Could you check a few things on this model? Use its own coordinates, in mm. Face numbers are marked on the shaded views. Give positions to 0.01 mm unless a question says otherwise; leave off trailing zeros. Order: outer loops, then holes, each group sorted by start corner. A loop starts at its lowest first (then second) coordinate and runs counter-clockwise, first axis right, second up.
(1) If I drill on probe 1 along Y at (x, z) = (121, 39); probe 2 along Z at (x, y) = (59.5, 113.5); probe 3 along X at (y, z) = (58.5, 81), over which ranges is the centre line in solid material (lowest first)?
(2) Imagine slicing it at B-B, the plane x = 42. Write out the boundary of the cut face in (y, z), then the cut area to 3 significant figures.
(3) Will these pins go through, and if not, where does the flat tip stop? pin 1 (7 mm diameter, centred on x = 111.5, y = -4, fed in from +Z); pin 2 (7 mm diameter, centred on x = 118, y = -2.5, fed in from -Z); pin 3 (1 mm diameter, centred on x = 81.5, z = 35, fed in from -Y); pin 4 (2 mm diameter, centred on x = 114.5, y = 70, fed in from +Z).
(4) If we mould it in two halves opening along X, with no side actions, what happens to the marked faces 1, 2, 3 and 4? For each: released by +X, released by -X, zero draft, split by the parting line, or undercut.
(5) Imagine slicing it at D-D, the plane z = 81.5. Write out the boundary of the cut face in (x, y), then the cut area to 3 significant figures.
(6) Imagine slicing it at C-C, the plane y = 35. Write out the boundary of the cut face in (x, z), then the cut area to 3 significant figures.
(7) Imagine slicing it at A-A, the plane z = 43.5. Write out the boundary of the cut face in (x, y), then the cut area to 3 significant figures.
from build123d import *

# Parameters (mm, degrees)
F0_W     = 152.4
F0_H     = 88.9
F1_DEPTH = 140.97
F2_R     = 12.7
F3_DEPTH = 12.7
F4_R     = 44.45
F5_DEPTH = 12.7
F6_R     = 31.75
F7_DEPTH = 12.7
F6_W     = 30.967094
F6_H     = 16.394339
F6_W_2   = 19.733936
F6_H_2   = 9.411566
F8_DEPTH = 6.35


with BuildPart() as f1:
    # F0 (on Front) → F1 (new body)
    with BuildSketch(Plane.XZ):
        with Locations((76.2, 44.45)):
            Rectangle(F0_W, F0_H)
    extrude(amount=-F1_DEPTH)

    # F2 (on face) → F3 (cut)
    with BuildSketch(Plane(origin=(0, 140.97, 0), x_dir=(-1, 0, 0), z_dir=(0, 1, 0))):
        with Locations((-133.2082, 19.652179)):
            Circle(F2_R)
    extrude(amount=-F3_DEPTH, mode=Mode.SUBTRACT)

    # F4 (on face) → F5 (cut)
    with BuildSketch(Plane.XY.offset(88.9)):
        with Locations((74.677013, 72.679326)):
            Circle(F4_R)
    extrude(amount=-F5_DEPTH, mode=Mode.SUBTRACT)

    # F6 (on face) → F7 (cut)
    with BuildSketch(Plane.XZ):
        with Locations((36.581997, 45.666065)):
            Circle(F6_R)
    extrude(amount=-F7_DEPTH, mode=Mode.SUBTRACT)

    # F6 (on face) → F8 (join)
    with BuildSketch(Plane.XZ):
        with Locations((114.606928, 71.168374)):
            Rectangle(F6_W, F6_H)
        with Locations((114.75873, 51.282644)):
            Rectangle(F6_W_2, F6_H_2)
    extrude(amount=F8_DEPTH)


solid = f1.part
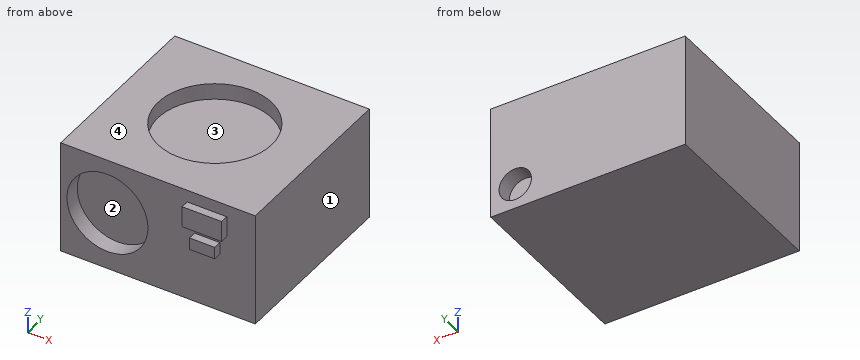
Answer block:
1. probe 1: y = 0 to 140.97
1. probe 2: z = 0 to 76.2
1. probe 3: x = 0 to 32.55, 116.8 to 152.4
2. outline: (0, 0) - (140.97, 0) - (140.97, 88.9) - (102.81, 88.9) - (102.81, 76.2) - (42.55, 76.2) - (42.55, 88.9) - (0, 88.9) - (0, 76.95) - (12.7, 76.95) - (12.7, 14.38) - (0, 14.38) - close
2. area: 11,000 mm2
3. pin 1: stops at z = 79.37
3. pin 2: stops at z = 0
3. pin 3: stops at y = 0
3. pin 4: stops at z = 76.2
4. face 1: released by +X
4. face 2: undercut
4. face 3: undercut
4. face 4: zero draft
5. outline: (0, 0) - (152.4, 0) - (152.4, 140.97) - (0, 140.97) - close; hole circle Ø88.9 at (74.68, 72.68)
5. area: 15,300 mm2
6. outline: (0, 0) - (152.4, 0) - (152.4, 88.9) - (98.26, 88.9) - (98.26, 76.2) - (51.1, 76.2) - (51.1, 88.9) - (0, 88.9) - close
6. area: 12,900 mm2
7. outline: (0, 0) - (4.91, 0) - (4.91, 12.7) - (68.26, 12.7) - (68.26, 0) - (152.4, 0) - (152.4, 140.97) - (0, 140.97) - close
7. area: 20,700 mm2
